```python
from build123d import *

# Parameters (mm, degrees)
MAIN_DEPTH          = 40
SKETCH11_W          = 100
SKETCH11_H          = 8
BOSS_EXTRUDE1_DEPTH = 80
FILLET1_R           = 40
SKETCH12_R          = 2.2
CUT_EXTRUDE1_DEPTH  = 162.365552125
SKETCH13_R          = 3.75
CUT_EXTRUDE2_DEPTH  = 4.5
CUT_EXTRUDE3_START  = 13
SKETCH14_W          = 80
SKETCH14_H          = 214.313708498
CUT_EXTRUDE3_DEPTH  = 7
CUT_EXTRUDE4_START  = 1
CUT_EXTRUDE4_DEPTH  = 135.291427387
FILLET2_R           = 10


with BuildPart() as part:
    # Sketch2 → Main (new, symmetric)
    with BuildSketch(Plane(origin=(0, 0, 0), x_dir=(0, 0, -1), z_dir=(1, 0, 0))):
        Polygon((-89, 0), (89, 0), (101.5, 12.5), (107.156854249, 6.843145751), (92.313708499, -8), (-92.313708499, -8), (-107.156854249, 6.843145751), (-101.5, 12.5), align=None)
    extrude(amount=MAIN_DEPTH, both=True)

    # Sketch11 → Boss-Extrude1 (add)
    with BuildSketch(Plane(origin=(40, 0, 0), x_dir=(0, 0, -1), z_dir=(1, 0, 0))):
        with Locations((0, -4)):
            Rectangle(SKETCH11_W, SKETCH11_H)
    extrude(amount=BOSS_EXTRUDE1_DEPTH)

    # Fillet1
    fillet1_edges = [part.edges().sort_by_distance(p)[0] for p in [
        (120, -4, -50),
        (40, -4, -50),
        (40, -4, 50),
        (120, -4, 50),
    ]]
    fillet(fillet1_edges, radius=FILLET1_R - 0.0001)  # a hair under: the kernel refuses the full size

    # Sketch12 → Cut-Extrude1 (cut, through all)
    with BuildSketch(Plane(origin=(0, 0, 0), x_dir=(1, 0, 0), z_dir=(0, 1, 0))):
        with Locations(Location((-10.606601718, 10.606601718, 0), (0, 0, 270))):
            Circle(SKETCH12_R)
        with Locations(Location((10.606601718, 10.606601718, 0), (0, 0, 270))):
            Circle(SKETCH12_R)
        with Locations(Location((10.606601718, -10.606601718, 0), (0, 0, 270))):
            Circle(SKETCH12_R)
        with Locations(Location((-10.606601718, -10.606601718, 0), (0, 0, 270))):
            Circle(SKETCH12_R)
    extrude(amount=-CUT_EXTRUDE1_DEPTH, mode=Mode.SUBTRACT)

    # Sketch13 → Cut-Extrude2 (cut)
    with BuildSketch(Plane(origin=(0, 0, 0), x_dir=(1, 0, 0), z_dir=(0, 1, 0))):
        with Locations(Location((-10.606601718, 10.606601718, 0), (0, 0, 270))):
            Circle(SKETCH13_R)
        with Locations(Location((10.606601718, 10.606601718, 0), (0, 0, 270))):
            Circle(SKETCH13_R)
        with Locations(Location((10.606601718, -10.606601718, 0), (0, 0, 270))):
            Circle(SKETCH13_R)
        with Locations(Location((-10.606601718, -10.606601718, 0), (0, 0, 270))):
            Circle(SKETCH13_R)
    extrude(amount=-CUT_EXTRUDE2_DEPTH, mode=Mode.SUBTRACT)

    # Sketch14 → Cut-Extrude3 (cut)
    with BuildSketch(Plane(origin=(0, 0, 0), x_dir=(1, 0, 0), z_dir=(0, 1, 0)).offset(CUT_EXTRUDE3_START)):
        Rectangle(SKETCH14_W, SKETCH14_H)
    extrude(amount=-CUT_EXTRUDE3_DEPTH, mode=Mode.SUBTRACT)

    # Sketch15 → Cut-Extrude4 (cut, through all)
    with BuildSketch(Plane(origin=(40, 0, 0), x_dir=(0, 0, -1), z_dir=(1, 0, 0)).offset(CUT_EXTRUDE4_START)):
        Polygon((106.313708499, 6), (92.313708499, -8), (86.656854249, -8), (100.656854249, 6), align=None)
    cut_extrude4 = extrude(amount=-CUT_EXTRUDE4_DEPTH, mode=Mode.SUBTRACT)

    # Mirror1: Cut-Extrude4 across plane
    add(cut_extrude4.mirror(Plane.XY), mode=Mode.SUBTRACT)

    # Fillet2
    fillet2_edges = [part.edges().sort_by_distance(p)[0] for p in [
        (0.069972296, -8, 86.656854249),
        (0.069972296, -8, -86.656854249),
    ]]
    fillet(fillet2_edges, radius=FILLET2_R)


solid = part.part
```
The model under review builds one solid part; all positions refer to its coordinate system, in mm. A direction names the side the tool comes from. Coordinates: 2 decimals unless noted, no trailing zeros. Write each loop counter-clockwise with the first axis right and the second up, starting at its lowest first coordinate (ties: lowest second). Pieces come first, ordered by that corner, then holes. Notation, with made-up numbers: (70.5, -1) -> (114.5, -1) arc R10 ccw to (114.5, 18) -> close; hole circle Ø2 at (46, 85.5). An arc over 180 degrees is marked (long way). One line per item, written item: value. Start each with the question number.
Q1. Add section D-D, the plane z = 86. Give the boundary of the cut face in (x, y).
Q2. Add section B-B, the plane y = -2.25. Count the separate pieces of the cut face and the enclosed holes in it, then the cut area to 3 significant figures.
Q3. The part is to be moulded in two halves that separate along X. For faces 1 (the face through (107.972, -3.944, -38.594)), 2 (the face through (-11.95, -6.23, -12.35)), 3 (the face through (-1, 6, -98)), say which applies: +X half, -X half, draft (parallel to the pull), parting line (faces both ways), or undercut.
Q4. To check wall thickness, follow probe 1 along Y at (x, z) = (-30, -60.5); probe 2 along Z at (x, y) = (-11.5, 5); probe 3 along Z at (x, y) = (38, 2.5). State the ranges of each line that lie inside material, in increasing order.
Q5. Add section C-C, the plane z = -36. Give the boundary of the cut face in (x, y).
Q6. For faces 4 (the face through (11, -4.5, 13)), 5 (the face through (40, 2, 94)), 6 (the face through (-0.21, -7.26, 86.29)), list the 3-axis set-ups (+Z, -Z, +X, -X, +Y, -Y) from which the entire face can be reached by the end or side of a thin tool; tool diameter is ignored.
Q7. Clearance check with flat-ended pins moving along their axes: P1, Ø2.5, axis at x = -10.61, z = 10.61, coming from the +Y side; P2, Ø5, axis at y = -1.5, z = -60, coming from the +X side; P3, Ø7, axis at x = -10.61, z = -10.61, coming from the +Y side; P4, Ø1.5, axis at x = 48.5, z = 27.5, coming from the +Y side. State where each tip first meets the part, or that it passes through.
Q8. Add section A-A, the plane x = -21. Give the boundary of the cut face in (y, z), then the cut area to 3 significant figures.
Response:
1. outline: (-40, -7.37) -> (40.2, -7.37) -> (40.2, 0) -> (-40, 0) -> close
2. separate pieces: 1
2. enclosed holes: 4
2. area: 22,600 mm²
3. face 1: +X half
3. face 2: undercut
3. face 3: draft
4. probe 1: -8 to 0
4. probe 2: -99.66 to -94, 94 to 99.66
4. probe 3: -97.16 to -91.5, 91.5 to 97.16
5. outline: (-40, -8) -> (110.4, -8) -> (110.4, 0) -> (-40, 0) -> close
6. face 4: +Y
6. face 5: +Z, +X, +Y, -Y
6. face 6: +Z, +X, -X, -Y
7. P1: through
7. P2: x = 56.68
7. P3: y = -4.5
7. P4: y = 0
8. outline: (-8, -82.51) arc R10 ccw to (-5.07, -89.59) -> (6, -100.66) -> (6, -95) -> (0, -89) -> (0, 89) -> (6, 95) -> (6, 100.66) -> (-5.07, 89.59) arc R10 ccw to (-8, 82.51) -> close
8. area: 1,510 mm²
